```python
from build123d import *

# Parameters (mm, degrees)
BOSS_EXTRUDE1_DEPTH     = 40
SKETCH2_R               = 24
BOSS_EXTRUDE2_DEPTH     = 40
SKETCH3_R               = 24
BOSS_EXTRUDE3_DEPTH     = 40
SCALE1_SCALE            = 0.125
FILLET3_R               = 4
FILLET4_R               = 4
CUT_EXTRUDE1_DEPTH      = 38.275
CUT_EXTRUDE1_DEPTH_BACK = 6
CUT_EXTRUDE2_DEPTH      = 38.275
CUT_EXTRUDE2_DEPTH_BACK = 6
SKETCH6_R               = 1.5
BOSS_EXTRUDE4_DEPTH     = 5


with BuildPart() as part:
    # Sketch1 → Boss-Extrude1 (new body)
    with BuildSketch(Plane(origin=(0, 0, 0), x_dir=(1, 0, 0), z_dir=(0, 1, 0))):
        Polygon((-173.422280891, 480), (-173.422280891, 450), (-800, 450), (-800, -450), (-173.422280891, -450), (-173.422280891, -480), (800, -480), (800, 480), align=None)
    extrude(amount=-BOSS_EXTRUDE1_DEPTH)

    # Sketch2 → Boss-Extrude2 (add)
    with BuildSketch(Plane.XY.offset(480)):
        with BuildLine():
            Line((218, 0), (298, 0))
            Line((298, 0), (298, 100))
            ThreePointArc((298, 100), (258, 140), (218, 100))
            Line((218, 100), (218, 0))
        make_face()
        with Locations((258, 100)):
            Circle(SKETCH2_R, mode=Mode.SUBTRACT)
        with BuildLine():
            Line((650, 258.2), (650, 0))
            Line((650, 0), (730, 0))
            Line((730, 0), (730, 258.2))
            ThreePointArc((730, 258.2), (690, 298.2), (650, 258.2))
        make_face()
        with Locations((690, 258.2)):
            Circle(SKETCH2_R, mode=Mode.SUBTRACT)
        Polygon((650, 0), (298, 0), (218, 0), (-173.422280891, 0), (-173.422280891, -40), (800, -40), (800, 0), (730, 0), align=None)
    extrude(amount=-BOSS_EXTRUDE2_DEPTH)

    # Mirror1: part across plane


with BuildPart() as part_1:
    add(part.part)
    add(part.part.mirror(Plane.XY))

    # Sketch3 → Boss-Extrude3 (add)
    with BuildSketch(Plane.XY.offset(450)):
        with BuildLine():
            Line((-414, 0), (-334, 0))
            Line((-334, 0), (-334, 162.7))
            ThreePointArc((-334, 162.7), (-374, 202.7), (-414, 162.7))
            Line((-414, 162.7), (-414, 0))
        make_face()
        with Locations((-374, 162.7)):
            Circle(SKETCH3_R, mode=Mode.SUBTRACT)
        with BuildLine():
            Line((-264, 0), (-184, 0))
            Line((-184, 0), (-184, 162.7))
            ThreePointArc((-184, 162.7), (-224, 202.7), (-264, 162.7))
            Line((-264, 162.7), (-264, 0))
        make_face()
        with Locations((-224, 162.7)):
            Circle(SKETCH3_R, mode=Mode.SUBTRACT)
    boss_extrude3 = extrude(amount=-BOSS_EXTRUDE3_DEPTH)

    # Mirror2: Boss-Extrude3 across plane
    add(boss_extrude3.mirror(Plane.XY))


with BuildPart() as part_2:
    # Scale1: scaled about (22.22402446, -11.339866564, 0)
    add(part_1.part.scale(SCALE1_SCALE).moved(Location((19.446021402, -9.922383243, 0))))

    # Fillet3
    fillet3_edges = [part_2.edges().sort_by_distance(p)[0] for p in [
        (-32.303978598, -9.922383243, 53.75),
        (-13.553978598, -9.922383243, 53.75),
        (-32.303978598, -9.922383243, -53.75),
        (-13.553978598, -9.922383243, -53.75),
        (46.696021403, -9.922383243, 57.5),
        (100.696021403, -9.922383243, 57.5),
        (100.696021403, -9.922383243, -57.5),
        (46.696021403, -9.922383243, -57.5),
    ]]
    fillet(fillet3_edges, radius=FILLET3_R)

    # Fillet4
    fillet4_edges = [part_2.edges().sort_by_distance(p)[0] for p in [
        (-3.553978598, -9.922383243, -53.75),
        (-22.303978598, -9.922383243, -53.75),
        (56.696021403, -9.922383243, -57.5),
        (110.696021402, -9.922383243, -57.5),
        (110.696021402, -9.922383243, 57.5),
        (56.696021403, -9.922383243, 57.5),
        (-3.553978598, -9.922383243, 53.75),
        (-22.303978598, -9.922383243, 53.75),
    ]]
    fillet(fillet4_edges, radius=FILLET4_R)

    # Sketch4 → Cut-Extrude1 (cut, two sides)
    with BuildSketch(Plane(origin=(0, -9.922383244, 0), x_dir=(1, 0, 0), z_dir=(0, 1, 0))) as cut_extrude1_sk:
        with BuildLine():
            Line((-60.553978598, 45), (99.446021402, 45))
            ThreePointArc((99.446021402, 45), (106.517089214, 42.071067812), (109.446021402, 35))
            Line((109.446021402, 35), (109.446021402, -35))
            ThreePointArc((109.446021402, -35), (106.517089214, -42.071067812), (99.446021402, -45))
            Line((99.446021402, -45), (-60.553978598, -45))
            ThreePointArc((-60.553978598, -45), (-67.62504641, -42.071067812), (-70.553978598, -35))
            Line((-70.553978598, -35), (-70.553978598, 35))
            ThreePointArc((-70.553978598, 35), (-67.62504641, 42.071067812), (-60.553978598, 45))
        make_face()
    extrude(amount=CUT_EXTRUDE1_DEPTH, mode=Mode.SUBTRACT)
    extrude(cut_extrude1_sk.sketch, amount=-CUT_EXTRUDE1_DEPTH_BACK, mode=Mode.SUBTRACT)

    # Sketch5 → Cut-Extrude2 (cut, two sides)
    with BuildSketch(Plane(origin=(0, -9.922383244, 0), x_dir=(1, 0, 0), z_dir=(0, 1, 0))) as cut_extrude2_sk:
        Polygon((0, 0), (123.509842575, 0), (123.509842575, -66.212941814), (-94.641009198, -66.212941814), (-94.641009198, 0), align=None)
    extrude(amount=CUT_EXTRUDE2_DEPTH, mode=Mode.SUBTRACT)
    extrude(cut_extrude2_sk.sketch, amount=-CUT_EXTRUDE2_DEPTH_BACK, mode=Mode.SUBTRACT)

    # Sketch6 → Boss-Extrude4 (add)
    with BuildSketch(Plane.XY):
        with Locations((-75.553978598, -12.422383244)):
            Circle(SKETCH6_R)
        with Locations((114.446021402, -12.422383244)):
            Circle(SKETCH6_R)
    extrude(amount=BOSS_EXTRUDE4_DEPTH)


solid = part_2.part
```
The model under review builds one solid part; all positions refer to its coordinate system, in mm. A direction names the side the tool comes from. Coordinates: 2 decimals unless noted, no trailing zeros. Write each loop counter-clockwise with the first axis right and the second up, starting at its lowest first coordinate (ties: lowest second). Pieces come first, ordered by that corner, then holes. Notation, with made-up numbers: (47.5, 51) -> (61.5, 51) arc R4 cw to (61.5, 56) -> close; hole circle Ø7 at (80, -14.5). An arc over 180 degrees is marked (long way). One line per item, written item: value. Start each with the question number.
Q1. The part is to be moulded in two halves that separate along Y. For faces 1 (the face through (-30.3, 10.55, -53.78)), 2 (the face through (26, -14.922, -46)), 3 (the face through (72, -11, -60)), say which applies: +Y half, -Y half, draft (parallel to the pull), parting line (faces both ways), or undercut.
Q2. Add section B-B, the plane x = 88.5. Give the boundary of the cut face in (y, z), then the cut area to 3 significant figures.
Q3. To check wall thickness, follow probe 1 along Z at (x, y) = (32.5, -12.5); probe 2 along Y at (x, z) = (84.5, -54); probe 3 along Z at (x, y) = (101.5, 5.5). State the ranges of each line that lie inside material, in increasing order.
Q4. Add section A-A, the plane z = -5. Give the boundary of the cut face in (x, y).
Q5. Clearance check with flat-ended pins moving along their axes: P1, Ø6, axis at y = -9.5, z = -41.5, coming from the -X side; P2, Ø1.5, axis at y = -0.5, z = -53.5, coming from the +X side; P3, Ø4, axis at x = 26.5, y = -11.5, coming from the +Z side; P4, Ø4, axis at y = 0, z = -56.5, coming from the +X side. State where each tip first meets the part, or that it passes through.
Q6. For faces 4 (the face through (-9, 0, -51.25)), 5 (the face through (27, -9.922, -48)), 6 (the face through (106, 9, -55)), 7 (the face through (99.493, -8.782, -57.465)), 8 (the face through (109.446, -12, -18)), list the 3-axis set-ups (+Z, -Z, +X, -X, +Y, -Y) from which the entire face can be reached by the end or side of a thin tool; tool diameter is ignored.
Response:
1. face 1: undercut
1. face 2: -Y half
1. face 3: draft
2. outline: (-14.92, -60) -> (-9.92, -60) -> (-9.92, -45) -> (-14.92, -45) -> close
2. area: 75.0 mm²
3. probe 1: -60 to -45
3. probe 2: -14.92 to -9.92
3. probe 3: -60 to -55
4. outline: (-80.55, -14.92) -> (-70.55, -14.92) -> (-70.55, -9.92) -> (-80.55, -9.92) -> close; (109.45, -14.92) -> (119.45, -14.92) -> (119.45, -9.92) -> (109.45, -9.92) -> close
5. P1: x = -80.55
5. P2: x = -3.55
5. P3: z = -45
5. P4: x = 110.7
6. face 4: +Z, +X, -X, +Y
6. face 5: +Z, +Y
6. face 6: +Z, +X, +Y
6. face 7: +Z, -Z, +Y
6. face 8: +Z, +Y, -Y
